Verification items for the finished model (mm, model axes). Face numbers are marked on the shaded views. A direction names the side the tool comes from. Give positions to 0.01 mm unless a question says otherwise; leave off trailing zeros. Write each loop counter-clockwise with the first axis right and the second up, starting at its lowest first coordinate (ties: lowest second). Pieces come first, ordered by that corner, then holes. Notation, with made-up numbers: (73.5, -25) -> (104.5, -25) arc R10 cw to (104.5, -19) -> close; hole circle Ø4 at (15, 31.5). An arc over 180 degrees is marked (long way). Use one line per item in the form item = value. Start each with the question number.
(1) Set-up check for the marked faces 5 and 6: record each of +Z, -Z, +X, -X, +Y, -Y from which the full face is reachable in a straight line by a thin tool's end or side.
(2) Scan lines: L1, parallel to X at y = 1.5, z = -20.5; L2, parallel to X at y = 5.5, z = 4.5; L3, parallel to Z at x = -10.5, y = 7.5. Record each from-to range of solid material in increasing order.
(3) Section check C-C, the plane x = -21. Record the cut outline in (y, z), plus the area to 3 significant figures.
(4) Section check A-A, the plane y = 8. Record the cut outline in (x, z), plus the area to 3 significant figures.
(5) Release check for a two-part mould opening along Z. For the marked faces 1, 2, 3 and 4 record: pulls with the +Z half, pulls with the -Z half, needs draft (parallel to the pull), parting line crosses it, or undercut.
(6) Depth check by flat-ended pin: pin 1 Ø1.4 at (x, z) = (46, 19.5) entering from +Y; pin 2 Ø10 at (x, z) = (10, 0) entering from -Y; pin 3 Ø6 at (x, z) = (21.5, 9) entering from +Y. Enter the tip coordinate at first touch or a pass-through.
(7) Section check B-B, the plane z = -16. Record the cut outline in (x, y), plus the area to 3 significant figures.
(8) Section check D-D, the plane z = -2. Record the cut outline in (x, y).
from build123d import *
from OCP.BRepFilletAPI import BRepFilletAPI_MakeFillet

# Parameters (mm, degrees)
SKETCH2_W           = 102
SKETCH2_H           = 50
BOSS_EXTRUDE2_DEPTH = 2
SKETCH1_W           = 102
SKETCH1_H           = 50
SKETCH1_W_2         = 98
SKETCH1_H_2         = 46
BOSS_EXTRUDE1_DEPTH = 12
FILLET1_R1          = 2
FILLET1_R2          = 1
BOSS_EXTRUDE3_DEPTH = 3
SKETCH4_R           = 0.9
BOSS_EXTRUDE4_DEPTH = 4
SKETCH5_W           = 15
SKETCH5_H           = 4
SKETCH5_W_2         = 13
CUT_EXTRUDE1_DEPTH  = 10


with BuildPart() as part:
    # Sketch2 → Boss-Extrude2 (new body)
    with BuildSketch(Plane(origin=(0, 0, 0), x_dir=(1, 0, 0), z_dir=(0, 1, 0))):
        Rectangle(SKETCH2_W, SKETCH2_H)
    extrude(amount=BOSS_EXTRUDE2_DEPTH)

    # Sketch1 → Boss-Extrude1 (add)
    with BuildSketch(Plane(origin=(0, 0, 0), x_dir=(1, 0, 0), z_dir=(0, 1, 0))):
        Rectangle(SKETCH1_W, SKETCH1_H)
        Rectangle(SKETCH1_W_2, SKETCH1_H_2, mode=Mode.SUBTRACT)
    extrude(amount=BOSS_EXTRUDE1_DEPTH)

    # Fillet1: one fillet with a radius per group of edges: ONE call of the kernel's fillet builder (fillet() takes one radius for all edges)
    fillet1_edges_1 = [part.edges().sort_by_distance(p)[0] for p in [
        (51, 6, 25),
        (51, 6, -25),
        (-51, 6, -25),
        (-51, 6, 25),
    ]]
    fillet1_edges_2 = [part.edges().sort_by_distance(p)[0] for p in [
        (-49, 7, 23),
        (49, 7, 23),
        (49, 7, -23),
        (-49, 7, -23),
    ]]
    fillet1 = BRepFilletAPI_MakeFillet(part.part.solid().wrapped)
    for e in fillet1_edges_1:
        fillet1.Add(FILLET1_R1, e.wrapped)
    for e in fillet1_edges_2:
        fillet1.Add(FILLET1_R2, e.wrapped)
    add(Compound.cast(fillet1.Shape()), mode=Mode.REPLACE)

    # Sketch3 → Boss-Extrude3 (add)
    with BuildSketch(Plane(origin=(0, 2, 0), x_dir=(1, 0, 0), z_dir=(0, 1, 0))):
        with BuildLine():
            ThreePointArc((-44.75, 19.75), (-47.310660172, 20.810660172), (-46.25, 18.25))
            Line((-46.25, 18.25), (-46.25, 19.75))
            Line((-46.25, 19.75), (-44.75, 19.75))
        make_face()
        with BuildLine():
            Line((-46.25, 19.75), (-46.25, 18.25))
            ThreePointArc((-46.25, 18.25), (-45.189339828, 18.689339828), (-44.75, 19.75))
            Line((-44.75, 19.75), (-46.25, 19.75))
        make_face()
        with BuildLine():
            Line((-46.25, -18.25), (-46.25, -19.75))
            Line((-46.25, -19.75), (-44.75, -19.75))
            ThreePointArc((-44.75, -19.75), (-45.189339828, -18.689339828), (-46.25, -18.25))
        make_face()
        with BuildLine():
            Line((-44.75, -19.75), (-46.25, -19.75))
            Line((-46.25, -19.75), (-46.25, -18.25))
            ThreePointArc((-46.25, -18.25), (-47.310660172, -20.810660172), (-44.75, -19.75))
        make_face()
        with BuildLine():
            ThreePointArc((46.25, -18.25), (45.189339828, -18.689339828), (44.75, -19.75))
            Line((44.75, -19.75), (46.25, -19.75))
            Line((46.25, -19.75), (46.25, -18.25))
        make_face()
        with BuildLine():
            Line((46.25, -19.75), (44.75, -19.75))
            ThreePointArc((44.75, -19.75), (46.25, -21.25), (47.75, -19.75))
            ThreePointArc((47.75, -19.75), (47.310660172, -18.689339828), (46.25, -18.25))
            Line((46.25, -18.25), (46.25, -19.75))
        make_face()
        with BuildLine():
            ThreePointArc((44.75, 19.75), (45.189339828, 18.689339828), (46.25, 18.25))
            Line((46.25, 18.25), (46.25, 19.75))
            Line((46.25, 19.75), (44.75, 19.75))
        make_face()
        with BuildLine():
            Line((46.25, 19.75), (46.25, 18.25))
            ThreePointArc((46.25, 18.25), (47.310660172, 18.689339828), (47.75, 19.75))
            ThreePointArc((47.75, 19.75), (46.25, 21.25), (44.75, 19.75))
            Line((44.75, 19.75), (46.25, 19.75))
        make_face()
    extrude(amount=BOSS_EXTRUDE3_DEPTH)

    # Sketch4 → Boss-Extrude4 (add)
    with BuildSketch(Plane(origin=(0, 5, 0), x_dir=(1, 0, 0), z_dir=(0, 1, 0))):
        with Locations(Location((-46.25, 19.75, 0), (0, 0, 270))):
            Circle(SKETCH4_R)
        with Locations(Location((-46.25, -19.75, 0), (0, 0, 270))):
            Circle(SKETCH4_R)
        with Locations(Location((46.25, 19.75, 0), (0, 0, 270))):
            Circle(SKETCH4_R)
        with Locations(Location((46.25, -19.75, 0), (0, 0, 270))):
            Circle(SKETCH4_R)
    extrude(amount=BOSS_EXTRUDE4_DEPTH)

    # Sketch5 → Cut-Extrude1 (cut)
    with BuildSketch(Plane(origin=(0, 2, 0), x_dir=(1, 0, 0), z_dir=(0, 1, 0))):
        with Locations((-23.5, 19)):
            Rectangle(SKETCH5_W, SKETCH5_H)
        with Locations((37.5, 17)):
            Rectangle(SKETCH5_W_2, SKETCH5_H)
    extrude(amount=-CUT_EXTRUDE1_DEPTH, mode=Mode.SUBTRACT)


solid = part.part
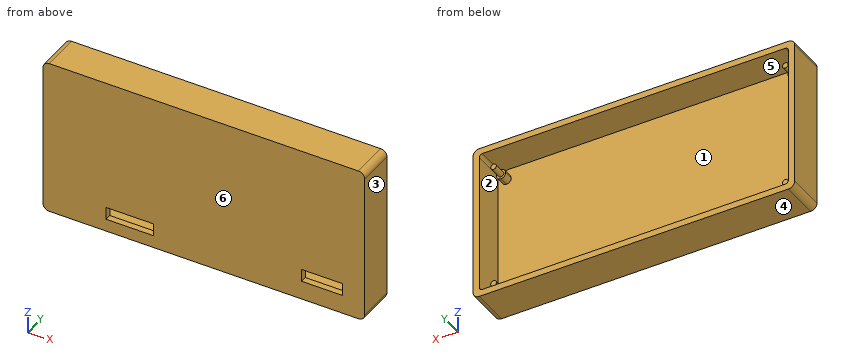
Completed:
q1.face_5 = +Y
q1.face_6 = +Z, -Z, +X, -X, -Y
q2.L1 = -51 to -31, -16 to 51
q2.L2 = -51 to -49, 49 to 51
q2.L3 = -25 to -23, 23 to 25
q3.outline = (0, -25) -> (12, -25) -> (12, -23) -> (2, -23) -> (2, -21) -> (0, -21) -> close; (0, -17) -> (2, -17) -> (2, 23) -> (12, 23) -> (12, 25) -> (0, 25) -> close
q3.area = 132 mm²
q4.outline = (-51, -23) arc R2 ccw to (-49, -25) -> (49, -25) arc R2 ccw to (51, -23) -> (51, 23) arc R2 ccw to (49, 25) -> (-49, 25) arc R2 ccw to (-51, 23) -> close; circle Ø1.8 at (-46.25, -19.75); circle Ø1.8 at (-46.25, 19.75); circle Ø1.8 at (46.25, -19.75); circle Ø1.8 at (46.25, 19.75); hole (-49, -22) arc R1 ccw to (-48, -23) -> (48, -23) arc R1 ccw to (49, -22) -> (49, 22) arc R1 ccw to (48, 23) -> (-48, 23) arc R1 ccw to (-49, 22) -> close
q4.area = 600 mm²
q5.face_1 = undercut
q5.face_2 = undercut
q5.face_3 = needs draft
q5.face_4 = pulls with the -Z half
q6.pin_1 = 9
q6.pin_2 = 0
q6.pin_3 = 2
q7.outline = (-51, 0) -> (31, 0) -> (31, 2) -> (-49, 2) -> (-49, 12) -> (-51, 12) -> close; (44, 0) -> (51, 0) -> (51, 12) -> (49, 12) -> (49, 2) -> (44, 2) -> close
q7.area = 218 mm²
q8.outline = (-51, 0) -> (51, 0) -> (51, 12) -> (49, 12) -> (49, 2) -> (-49, 2) -> (-49, 12) -> (-51, 12) -> close
